from build123d import *

# Parameters (mm, degrees)
F0_W     = 50.8
F0_H     = 31.75
F1_DEPTH = 31.75
F2_W     = 19.05
F2_H     = 19.05
F3_DEPTH = 50.8
F5_DEPTH = 25.4
F6_W     = 13.051277
F6_H     = 19.05
F7_DEPTH = 12.7


with BuildPart() as f1:
    # F0 (on Front) → F1 (new body)
    with BuildSketch(Plane.XZ):
        with Locations((25.4, 15.875)):
            Rectangle(F0_W, F0_H)
    extrude(amount=F1_DEPTH)

    # F2 (on face) → F3 (cut)
    with BuildSketch(Plane.YZ.offset(50.8)):
        with Locations((-22.225, 22.225)):
            Rectangle(F2_W, F2_H)
    extrude(amount=-F3_DEPTH, mode=Mode.SUBTRACT)

    # F4 (on face) → F5 (cut)
    with BuildSketch(Plane.XZ.offset(12.7)):
        Polygon((50.8, 31.75), (38.1, 31.75), (50.8, 12.7), align=None)
    extrude(amount=-F5_DEPTH, mode=Mode.SUBTRACT)

    # F6 (on face) → F7 (join)
    with BuildSketch(Plane.XZ.offset(12.7)):
        with Locations((25.109522, 22.225)):
            Rectangle(F6_W, F6_H)
    extrude(amount=F7_DEPTH)


solid = f1.part
Geometry check sheet. Reference: the model listing, model coordinates, mm. A direction names the side the tool comes from. Round coordinates to 2 decimals unless told otherwise and drop trailing zeros. Order: outer loops, then holes, each group sorted by start corner. A loop starts at its lowest first (then second) coordinate and runs counter-clockwise, first axis right, second up. Notation, with made-up numbers: (79, 40) - (92, 40) arc R24 cw to (92, 66) - close; hole circle Ø10 at (39.25, 60). An arc over 180 degrees is marked (long way). One line per question, with ' | ' between items. Start each with the question number.
(1) Thickness scan on L1, parallel to Y at x = 36, z = 15.5; L2, parallel to Y at x = 29, z = 26; L3, parallel to Z at x = 6, y = -18.5. Record the ranges inside material, lowest first. Write a range as [from, to].
(2) Access from +Z, -Z, +X, -X, +Y, -Y to the whole of each face (thin tool, end or side, straight path). Record for faces 1 (the flat face through (31.635, -19, 22)), 2 (the flat face through (25, -31.75, 6)), 3 (the flat face through (9, -12.7, 22)), 4 (the flat face through (25, -25.4, 22)), 5 (the flat face through (25, 0, 16)).
(3) Sectioned sample at B-B on x = 47.5. Record the cut outline in (y, z).
(4) Sectioned sample at C-C on z = 20. Record the cut outline in (x, y), and give its area (3 significant figures).
(5) Sectioned sample at D-D on y = -14. Record the cut outline in (x, z).
(6) Depth check by flat-ended pin: pin 1 Ø9.5 at (x, z) = (40, 25) entering from -Y; pin 2 Ø6.5 at (y, z) = (-19, 25) entering from -X; pin 3 Ø14 at (y, z) = (-17, 18) entering from +X; pin 4 Ø5 at (y, z) = (-8.5, 27) entering from +X. Enter the tip coordinate at first touch or a pass-through.
(7) Sectioned sample at A-A on y = -1.5. Record the cut outline in (x, z), and give its area (3 significant figures).
Conclusion:
1) L1: y = [-12.7, 0] | L2: y = [-25.4, 0] | L3: z = [0, 12.7]
2) face 1: +Z, +X, -Y | face 2: +Z, -Z, +X, -X, -Y | face 3: +Z, -X, -Y | face 4: +Z, +X, -X, -Y | face 5: +Z, -Z, +X, -X, +Y
3) outline: (-31.75, 0) - (0, 0) - (0, 17.65) - (-12.7, 17.65) - (-12.7, 12.7) - (-31.75, 12.7) - close
4) outline: (0, -12.7) - (18.58, -12.7) - (18.58, -25.4) - (31.64, -25.4) - (31.64, -12.7) - (45.93, -12.7) - (45.93, 0) - (0, 0) - close | area: 749 mm2
5) outline: (0, 0) - (50.8, 0) - (50.8, 12.7) - (31.64, 12.7) - (31.64, 31.75) - (18.58, 31.75) - (18.58, 12.7) - (0, 12.7) - close
6) pin 1: stops at y = -12.7 | pin 2: stops at x = 18.58 | pin 3: stops at x = 50.8 | pin 4: stops at x = 42.93
7) outline: (0, 0) - (50.8, 0) - (50.8, 12.7) - (38.1, 31.75) - (0, 31.75) - close | area: 1,490 mm2
